Read the model definition and answer for the solid it produces. Units are mm, in the model's axes. Face numbers are marked on the shaded views. A direction names the side the tool comes from. Give positions to 0.01 mm unless a question says otherwise; leave off trailing zeros. Write each loop counter-clockwise with the first axis right and the second up, starting at its lowest first coordinate (ties: lowest second). Pieces come first, ordered by that corner, then holes. Notation, with made-up numbers: (82, -2.5) -> (127, -2.5) arc R18 ccw to (127, 20.5) -> close; hole circle Ø3 at (-5, 52). An arc over 180 degrees is marked (long way). Answer as CSV lines item,"result". Start each with the question number.
1. A tool of negligible diameter and unlimited length cuts with its end or side. For the marked faces 1, 2 and 3, from which of +Z, -Z, +X, -X, +Y, -Y can it reach the whole face along a straight path? Write none if from no direction.
2. The part is cut by section C-C, the plane y = 3.7. Determine the outline of the cut face in (x, z), and give its area (3 significant figures).
3. The part is cut by section D-D, the plane x = 2.75. Determine the outline of the cut face in (y, z).
4. Find the intervals of material crossed by line 1 (Y direction, x = -1.75, z = 3.5); line 2 (Z direction, x = -0.5, y = 0.4); line 3 (Z direction, x = -1, y = 2.75), in increasing order.
5. The part is cut by section B-B, the plane z = 0. Determine the outline of the cut face in (x, y).
6. For a pull along X with two mould halves and no side action, classify the marked faces 4, 5, 6 and 7 as pulls with the +X half, pulls with the -X half, needs draft (parallel to the pull), parting line crosses it, or undercut.
7. The part is cut by section A-A, the plane x = 0. Determine the outline of the cut face in (y, z).
8. Given pin 1 (2 mm diameter, centred on y = 1.5, z = -1, fed in from +X); pin 2 (2 mm diameter, centred on x = -3.5, z = -2.5, fed in from -Y), each flat-ended and moving along its own axis, determine where each tip first touches the part or whether it passes through.
from build123d import *

# Parameters (mm, degrees)
SKETCH1_R           = 3.5
BOSS_EXTRUDE1_DEPTH = 4
BOSS_EXTRUDE2_START = -1
SKETCH2_R           = 4.5
SKETCH2_R_2         = 3.5
BOSS_EXTRUDE2_DEPTH = 1
SKETCH3_R           = 4.5
SKETCH3_R_2         = 3.5
BOSS_EXTRUDE4_DEPTH = 1


with BuildPart() as part:
    # Sketch1 → Boss-Extrude1 (new body)
    with BuildSketch(Plane(origin=(0, 0, 0), x_dir=(1, 0, 0), z_dir=(0, 1, 0))):
        with Locations(Location((0, 0, 0), (0, 0, 270))):
            Circle(SKETCH1_R)
        with BuildLine():
            Line((-1.5, 2), (-1.5, -2))
            ThreePointArc((-1.5, -2), (0, -2.5), (1.5, -2))
            Line((1.5, -2), (1.5, 2))
            ThreePointArc((1.5, 2), (0, 2.5), (-1.5, 2))
        make_face(mode=Mode.SUBTRACT)
    extrude(amount=BOSS_EXTRUDE1_DEPTH)

    # Sketch2 → Boss-Extrude2 (add)
    with BuildSketch(Plane(origin=(0, 4, 0), x_dir=(1, 0, 0), z_dir=(0, 1, 0)).offset(BOSS_EXTRUDE2_START)):
        with Locations(Location((0, 0, 0), (0, 0, 270))):
            Circle(SKETCH2_R)
        with Locations(Location((0, 0, 0), (0, 0, 270))):
            Circle(SKETCH2_R_2, mode=Mode.SUBTRACT)
    extrude(amount=BOSS_EXTRUDE2_DEPTH)

    # Sketch3 → Boss-Extrude4 (add)
    with BuildSketch(Plane.XZ):
        with Locations(Location((0, 0, 0), (0, 0, 90))):
            Circle(SKETCH3_R)
        with Locations(Location((0, 0, 0), (0, 0, 270))):
            Circle(SKETCH3_R_2, mode=Mode.SUBTRACT)
    extrude(amount=-BOSS_EXTRUDE4_DEPTH)


solid = part.part
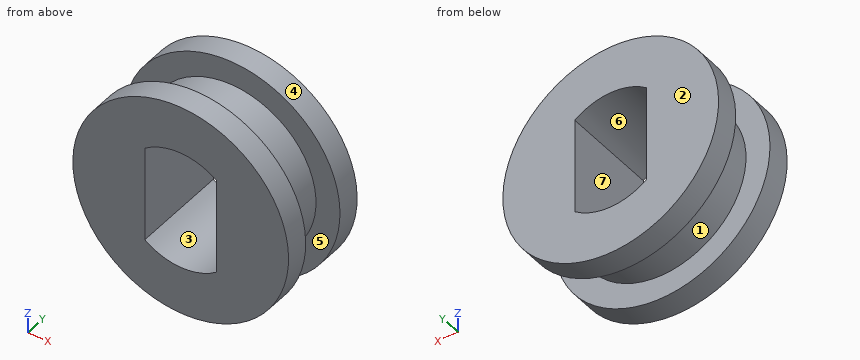
Results found:
1,face 1,"none"
1,face 2,"+Z, -Z, +X, -X, +Y"
1,face 3,"+Y, -Y"
2,outline,"circle Ø9 at (0, 0); hole (-1.5, -2) arc R2.5 ccw to (1.5, -2) -> (1.5, 2) arc R2.5 ccw to (-1.5, 2) -> close"
2,area,"49.6 mm²"
3,outline,"(0, -3.56) -> (1, -3.56) -> (1, -2.17) -> (3, -2.17) -> (3, -3.56) -> (4, -3.56) -> (4, 3.56) -> (3, 3.56) -> (3, 2.17) -> (1, 2.17) -> (1, 3.56) -> (0, 3.56) -> close"
4,line 1,"y = 0 to 1, 3 to 4"
4,line 2,"z = -4.47 to -2.45, 2.45 to 4.47"
4,line 3,"z = -3.35 to -2.29, 2.29 to 3.35"
5,outline,"(-4.5, 0) -> (-1.5, 0) -> (-1.5, 4) -> (-4.5, 4) -> (-4.5, 3) -> (-3.5, 3) -> (-3.5, 1) -> (-4.5, 1) -> close; (1.5, 0) -> (4.5, 0) -> (4.5, 1) -> (3.5, 1) -> (3.5, 3) -> (4.5, 3) -> (4.5, 4) -> (1.5, 4) -> close"
6,face 4,"parting line crosses it"
6,face 5,"needs draft"
6,face 6,"undercut"
6,face 7,"undercut"
7,outline,"(0, -4.5) -> (1, -4.5) -> (1, -3.5) -> (3, -3.5) -> (3, -4.5) -> (4, -4.5) -> (4, -2.5) -> (0, -2.5) -> close; (0, 2.5) -> (4, 2.5) -> (4, 4.5) -> (3, 4.5) -> (3, 3.5) -> (1, 3.5) -> (1, 4.5) -> (0, 4.5) -> close"
8,pin 1,"stops at x = 4.5"
8,pin 2,"stops at y = 0"
